For this review, take the finished solid that the model builds, in its own axes (mm). Face numbers are marked on the shaded views. Coordinates: 2 decimals unless noted, no trailing zeros. Order: outer loops, then holes, each group sorted by start corner. A loop starts at its lowest first (then second) coordinate and runs counter-clockwise, first axis right, second up.
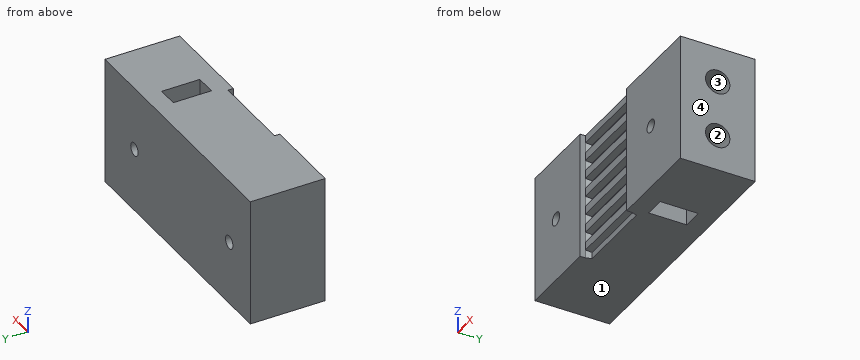
from build123d import *

# Parameters (mm, degrees)
SKETCH1_W           = 68.896006058
SKETCH1_H           = 34.135361424
BOSS_EXTRUDE1_DEPTH = 20
CUT_EXTRUDE1_REACH  = 36.135
SKETCH2_W           = 22.032289941
SKETCH2_H           = 1.4
SKETCH7_R           = 3.25
CUT_EXTRUDE4_DEPTH  = 30
CUT_EXTRUDE5_REACH  = 22
SKETCH8_R           = 1.75
SKETCH9_W           = 5.5
SKETCH9_H           = 10.2
CUT_EXTRUDE6_DEPTH  = 35.135361425
SKETCH10_W          = 22.032289941
SKETCH10_H          = 2.8
CUT_EXTRUDE7_DEPTH  = 1.5
CUT_EXTRUDE7_TAPER  = 20
LPATTERN1_COUNT     = 7
LPATTERN1_PITCH     = 5


with BuildPart() as part:
    # Sketch1 → Boss-Extrude1 (new body)
    with BuildSketch(Plane(origin=(0, 0, 0), x_dir=(1, 0, 0), z_dir=(0, 1, 0))):
        Rectangle(SKETCH1_W, SKETCH1_H)
    extrude(amount=BOSS_EXTRUDE1_DEPTH)

    # Sketch2 → Cut-Extrude1 (cut, up to next)
    with BuildSketch(Plane(origin=(0, 0, -17.067680712), x_dir=(-1, 0, 0), z_dir=(0, 0, -1)), mode=Mode.PRIVATE) as cut_extrude1_sk1:
        with Locations((1.973306179, 0.7)):
            Rectangle(SKETCH2_W, SKETCH2_H)
    cut_extrude1_tool1 = extrude(cut_extrude1_sk1.sketch, amount=-CUT_EXTRUDE1_REACH, mode=Mode.PRIVATE) & part.part
    add(cut_extrude1_tool1.solids().sort_by_distance((-1.973306, 0.7, -17.067681))[0], mode=Mode.SUBTRACT)

    # Sketch7 → Cut-Extrude4 (cut)
    with BuildSketch(Plane(origin=(34.448003029, 0, 0), x_dir=(0, 0, -1), z_dir=(1, 0, 0))):
        with Locations((-7.5, 10)):
            Circle(SKETCH7_R)
        with Locations((7.5, 10)):
            Circle(SKETCH7_R)
    extrude(amount=-CUT_EXTRUDE4_DEPTH, mode=Mode.SUBTRACT)

    # Sketch8 → Cut-Extrude5 (cut, up to next)
    with BuildSketch(Plane.XZ, mode=Mode.PRIVATE) as cut_extrude5_sk1:
        with Locations((-24.448003029, 0)):
            Circle(SKETCH8_R)
    cut_extrude5_tool1 = extrude(cut_extrude5_sk1.sketch, amount=-CUT_EXTRUDE5_REACH, mode=Mode.PRIVATE) & part.part
    add(cut_extrude5_tool1.solids().sort_by_distance((-24.448003, 0, 0))[0], mode=Mode.SUBTRACT)
    # Sketch8 → Cut-Extrude5 (cut, up to next)
    with BuildSketch(Plane.XZ, mode=Mode.PRIVATE) as cut_extrude5_sk2:
        with Locations((20.448003029, 0)):
            Circle(SKETCH8_R)
    cut_extrude5_tool2 = extrude(cut_extrude5_sk2.sketch, amount=-CUT_EXTRUDE5_REACH, mode=Mode.PRIVATE) & part.part
    add(cut_extrude5_tool2.solids().sort_by_distance((20.448003, 0, 0))[0], mode=Mode.SUBTRACT)

    # Sketch9 → Cut-Extrude6 (cut, through all)
    with BuildSketch(Plane(origin=(0, 0, -17.067680712), x_dir=(-1, 0, 0), z_dir=(0, 0, -1))):
        with Locations((-13.475884112, 10)):
            Rectangle(SKETCH9_W, SKETCH9_H)
    extrude(amount=-CUT_EXTRUDE6_DEPTH, mode=Mode.SUBTRACT)

    # Sketch10 → Cut-Extrude7 (cut)
    with BuildSketch(Plane.XZ.offset(-1.4)):
        with Locations((-1.973306179, 13.755042689)):
            Rectangle(SKETCH10_W, SKETCH10_H)
    cut_extrude7 = extrude(amount=-CUT_EXTRUDE7_DEPTH, taper=CUT_EXTRUDE7_TAPER, mode=Mode.SUBTRACT)

    # LPattern1: Cut-Extrude7 ×7
    with Locations(*[(0, 0, -i * LPATTERN1_PITCH) for i in range(1, LPATTERN1_COUNT)]):
        add(cut_extrude7, mode=Mode.SUBTRACT)


solid = part.part
1. The part is to be moulded in two halves that separate along Z. For the marked faces 1, 2, 3 and 4, say which applies: +Z half, -Z half, draft (parallel to the pull), parting line (faces both ways), or undercut.
Answer below:
face 1: -Z half
face 2: undercut
face 3: undercut
face 4: draft
2. Take a section at B-B, the plane x = 14. Give the boundary of the cut face in (y, z), plus the area to 3 significant figures.
Answer below:
outline: (0, -17.07) - (4.9, -17.07) - (4.9, 17.07) - (0, 17.07) - close; (15.1, -17.07) - (20, -17.07) - (20, 17.07) - (15.1, 17.07) - close
area: 335 mm2
3. Take a section at A-A, the plane y = 10. Give the boundary of the cut face in (x, z), plus the area to 3 significant figures.
Answer below:
outline: (-34.45, -17.07) - (10.73, -17.07) - (10.73, -10.75) - (4.45, -10.75) - (4.45, -4.25) - (10.73, -4.25) - (10.73, 4.25) - (4.45, 4.25) - (4.45, 10.75) - (10.73, 10.75) - (10.73, 17.07) - (-34.45, 17.07) - close; (16.23, -17.07) - (34.45, -17.07) - (34.45, -10.75) - (16.23, -10.75) - close; (16.23, -4.25) - (34.45, -4.25) - (34.45, 4.25) - (16.23, 4.25) - close; (16.23, 10.75) - (34.45, 10.75) - (34.45, 17.07) - (16.23, 17.07) - close; hole circle Ø3.5 at (-24.45, 0); hole circle Ø3.5 at (20.45, 0)
area: 1,830 mm2
4. Clearance check with flat-ended pins moving along their axes: pin 1 Ø3 at (y, z) = (11.5, -7.5) entering from +X; pin 2 Ø5 at (y, z) = (9.5, 9) entering from +X; pin 3 Ø1.8 at (x, z) = (-3, -8.5) entering from -Y; pin 4 Ø0.9 at (x, z) = (0.5, 9) entering from -Y. State where each tip first meets the part, or that it passes through.
Answer below:
pin 1: stops at x = 4.45
pin 2: stops at x = 34.45
pin 3: stops at y = 1.4
pin 4: stops at y = 2.9
5. To check wall thickness, follow L1, parallel to Z at x = 23, y = 9.75; L2, parallel to X at y = 11, z = 15.5; L3, parallel to Z at x = -24.5, y = 17.25. State the ranges of each line that lie inside material, in increasing order.
Answer below:
L1: z = -17.07 to -10.74, -4.26 to 4.26, 10.74 to 17.07
L2: x = -34.45 to 10.73, 16.23 to 34.45
L3: z = -17.07 to -1.75, 1.75 to 17.07
